from build123d import *

# Parameters (mm, degrees)
ESBO_O4_W                = 76
ESBO_O4_H                = 76
RESSALTO_EXTRUS_O2_DEPTH = 45


with BuildPart() as part:
    # Esboço4 → Ressalto-extrusão2 (new body)
    with BuildSketch(Plane.XY):
        Rectangle(ESBO_O4_W, ESBO_O4_H)
    extrude(amount=RESSALTO_EXTRUS_O2_DEPTH)

    # Esboço5 → Corte-Revolução2 (revolve, cut)
    with BuildSketch(Plane(origin=(0, 0, 0), x_dir=(0, 0, -1), z_dir=(1, 0, 0))):
        with BuildLine():
            Line((-104.6568392, 0), (-51.757946877, 0))
            ThreePointArc((-51.757946877, 0), (0, 51.757946877), (51.757946877, 0))
            Line((51.757946877, 0), (104.6568392, 0))
            ThreePointArc((104.6568392, 0), (0, 104.6568392), (-104.6568392, 0))
        make_face()
    revolve(axis=Axis((0, 0, 104.6568392), (0, 0, -1)), mode=Mode.SUBTRACT)


solid = part.part
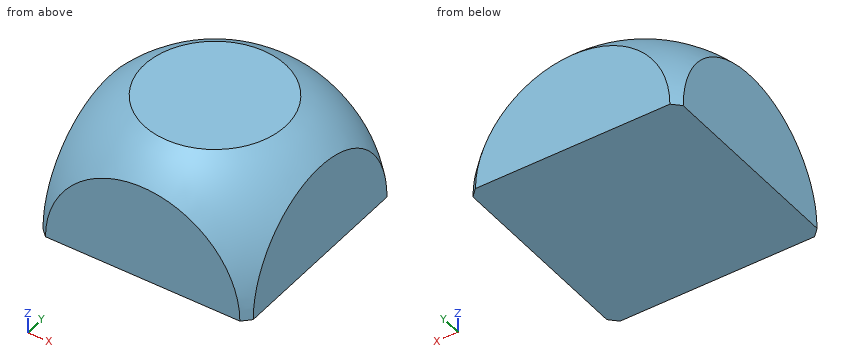
Build history of the part. All positions in model axes, mm. Round coordinates to 2 decimals unless told otherwise and drop trailing zeros. Write each loop counter-clockwise with the first axis right and the second up, starting at its lowest first coordinate (ties: lowest second). Pieces come first, ordered by that corner, then holes. Notation, with made-up numbers: (-26, -17.5) - (-22, -17.5) arc R16 cw to (-22, -3.5) - close; hole circle Ø9 at (46.25, 20.25). An arc over 180 degrees is marked (long way). One line per question, with ' | ' between items.
1. Band-saw the part on C-C, the plane x = 12.5. Write the cut outline in (y, z), and give its area (3 significant figures).
Results are:
outline: (-38, 0) - (38, 0) - (38, 32.84) arc R50.23 ccw to (22.31, 45) - (-22.31, 45) arc R50.23 ccw to (-38, 32.84) - close | area: 3,260 mm^2
2. Band-saw the part on B-B, the plane y = -0.5. Write the cut outline in (x, z), and give its area (3 significant figures).
Results are:
outline: (-38, 0) - (38, 0) - (38, 35.14) arc R51.76 ccw to (25.57, 45) - (-25.57, 45) arc R51.76 ccw to (-38, 35.14) - close | area: 3,310 mm^2
3. Drill centre lines: line 1 along Y through (x, z) = (-30, 33.5); line 2 along Z through (x, y) = (31, -14.5); line 3 along X through (y, z) = (10.5, 36). Where is each one in solid material? Low to high. Write a range as from..to.
Results are:
line 1: -25.62..25.62 | line 2: 0..38.83 | line 3: -35.67..35.67
4. Band-saw the part on A-A, the plane z = 32. Write the cut outline in (x, y), and give its area (3 significant figures).
Results are:
outline: (-38, -14.52) arc R40.68 ccw to (-14.52, -38) - (14.52, -38) arc R40.68 ccw to (38, -14.52) - (38, 14.52) arc R40.68 ccw to (14.52, 38) - (-14.52, 38) arc R40.68 ccw to (-38, 14.52) - close | area: 4,990 mm^2
5. Drop flat-ended pins along their axis: pin 1 Ø4 at (x, z) = (24, 37) entering from +Y; pin 2 Ø3 at (y, z) = (1.5, 38.5) entering from +X; pin 3 Ø5 at (x, z) = (-20.5, 34) entering from -Y. Give the stop position or say it passes through.
Results are:
pin 1: y = 30.1 | pin 2: x = 36.16 | pin 3: y = -35.98
6. Band-saw the part on D-D, the plane z = 20. Write the cut outline in (x, y), and give its area (3 significant figures).
Results are:
outline: (-38, -28.89) arc R47.74 ccw to (-28.89, -38) - (28.89, -38) arc R47.74 ccw to (38, -28.89) - (38, 28.89) arc R47.74 ccw to (28.89, 38) - (-28.89, 38) arc R47.74 ccw to (-38, 28.89) - close | area: 5,630 mm^2
